```python
from build123d import *

# Parameters (mm, degrees)
F0_W     = 76.2
F0_H     = 38.1
F1_DEPTH = 2.54
F2_R     = 4.402581
F3_DEPTH = 21.082
F5_DEPTH = 3.81


with BuildPart() as f1:
    # F0 (on Top) → F1 (new body)
    with BuildSketch(Plane.XY):
        with Locations((-22.33921, -2.823238)):
            Rectangle(F0_W, F0_H)
    extrude(amount=F1_DEPTH)

    # F2 (on face) → F3 (cut)
    with BuildSketch(Plane.XY.offset(2.54)):
        with Locations((8.346367, 0)):
            Circle(F2_R)
    extrude(amount=-F3_DEPTH, mode=Mode.SUBTRACT)

    # F4 (on face) → F5 (join)
    with BuildSketch(Plane.XY.offset(2.54)):
        with BuildLine():
            Line((-33.514785, 11.699406), (-35.571453, 1.141185))
            Line((-35.571453, 1.141185), (-23.946188, 6.15845))
            ThreePointArc((-23.946188, 6.15845), (-25.975231, 13.68694), (-33.514785, 11.699406))
        make_face()
        with BuildLine():
            Line((-35.571453, 1.141185), (-26.47813, -4.604892))
            ThreePointArc((-26.47813, -4.604892), (-19.860057, -0.482237), (-23.946188, 6.15845))
            Line((-23.946188, 6.15845), (-35.571453, 1.141185))
        make_face()
        with BuildLine():
            Line((-35.571453, 1.141185), (-35.112303, -11.512231))
            ThreePointArc((-35.112303, -11.512231), (-27.360523, -12.351928), (-26.47813, -4.604892))
            Line((-26.47813, -4.604892), (-35.571453, 1.141185))
        make_face()
        with BuildLine():
            Line((-40.746415, -10.414745), (-35.571453, 1.141185))
            Line((-35.571453, 1.141185), (-46.156678, -0.771649))
            ThreePointArc((-46.156678, -0.771649), (-48.246604, -8.283465), (-40.746415, -10.414745))
        make_face()
        with BuildLine():
            Line((-46.156678, -0.771649), (-35.571453, 1.141185))
            Line((-35.571453, 1.141185), (-44.463545, 10.155088))
            ThreePointArc((-44.463545, 10.155088), (-50.743462, 5.533635), (-46.156678, -0.771649))
        make_face()
        with BuildLine():
            Line((-44.463545, 10.155088), (-35.571453, 1.141185))
            Line((-35.571453, 1.141185), (-33.514785, 11.699406))
            ThreePointArc((-33.514785, 11.699406), (-34.841828, 14.557803), (-37.515037, 16.226762))
            Line((-37.515037, 16.226762), (-40.454786, 16.226762))
            ThreePointArc((-40.454786, 16.226762), (-43.598668, 13.94327), (-44.463545, 10.155088))
        make_face()
    extrude(amount=F5_DEPTH)


solid = f1.part
```
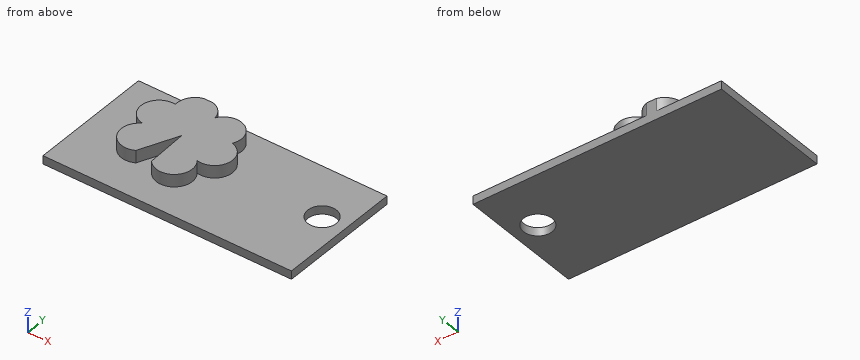
Build history of the part. All positions in model axes, mm. Round coordinates to 2 decimals unless told otherwise and drop trailing zeros. Write each loop counter-clockwise with the first axis right and the second up, starting at its lowest first coordinate (ties: lowest second). Pieces come first, ordered by that corner, then holes. Notation, with made-up numbers: (79, 7) - (98, 7) arc R31 ccw to (98, 45) - close; hole circle Ø3 at (15, -17). An arc over 180 degrees is marked (long way). Write each question's results on one line, items separated by ' | '. Start each with the question number.
Item 1: Saw through at D-D (x = -42.5). Write the cut outline in (y, z).
Item 2: Wall check: L1, parallel to Z at x = -17, y = 5.5; L2, parallel to Y at x = 7.5, z = 1; L3, parallel to X at y = -10, z = 5.25. Give the ranges that are in metal, low to high. Write a range as [from, to].
Item 3: Saw through at B-B (x = 6.5). Write the cut outline in (y, z).
Item 4: Saw through at C-C (z = 1.75). Write the cut outline in (x, y).
Item 5: Saw through at A-A (y = 0). Write the cut outline in (x, z), and give its area (3 significant figures).
Results are:
1) outline: (-21.87, 0) - (16.23, 0) - (16.23, 2.54) - (15.16, 2.54) - (15.16, 6.35) - (-11.03, 6.35) - (-11.03, 2.54) - (-21.87, 2.54) - close
2) L1: z = [0, 2.54] | L2: y = [-21.87, -4.32], [4.32, 16.23] | L3: x = [-46.74, -40.56], [-35.17, -25.65]
3) outline: (-21.87, 0) - (-4, 0) - (-4, 2.54) - (-21.87, 2.54) - close; (4, 0) - (16.23, 0) - (16.23, 2.54) - (4, 2.54) - close
4) outline: (-60.44, -21.87) - (15.76, -21.87) - (15.76, 16.23) - (-60.44, 16.23) - close; hole circle Ø8.81 at (8.35, 0)
5) outline: (-60.44, 0) - (3.94, 0) - (3.94, 2.54) - (-19.77, 2.54) - (-19.77, 6.35) - (-35.53, 6.35) - (-35.53, 2.54) - (-36.08, 2.54) - (-36.08, 6.35) - (-48.21, 6.35) - (-48.21, 2.54) - (-60.44, 2.54) - close; (12.75, 0) - (15.76, 0) - (15.76, 2.54) - (12.75, 2.54) - close | area: 277 mm²
